from build123d import *

# Parameters (mm, degrees)
SKETCH1_R               = 2
BOSS_EXTRUDE1_DEPTH     = 2
FILLET1_R               = 7
SKETCH2_R               = 1.5
BOSS_EXTRUDE2_DEPTH     = 2.2
SKETCH3_R               = 1
BOSS_EXTRUDE3_DEPTH     = 2
SKETCH4_W               = 2
SKETCH4_H               = 15
BOSS_EXTRUDE4_DEPTH     = 7
FILLET3_START           = -3
FILLET3_DEPTH           = 6
FILLET3_2_DEPTH         = 2
FILLET3_START_2         = 1
FILLET3_3_DEPTH         = 2
CUT_EXTRUDE1_DEPTH      = 47.08088663
CUT_EXTRUDE1_DEPTH_BACK = 47.08088663
SKETCH5_R               = 2


with BuildPart() as part:
    # Sketch1 → Boss-Extrude1 (new body)
    with BuildSketch(Plane(origin=(0, 0, 0), x_dir=(1, 0, 0), z_dir=(0, 1, 0))):
        Polygon((-15, 0), (15, 0), (24.948794511, 37.5), (-24.948794511, 37.5), align=None)
        with Locations(Location((10, 26, 0), (0, 0, 270))):
            Circle(SKETCH1_R, mode=Mode.SUBTRACT)
        with Locations(Location((10, 6, 0), (0, 0, 270))):
            Circle(SKETCH1_R, mode=Mode.SUBTRACT)
        with Locations(Location((-10, 6, 0), (0, 0, 90))):
            Circle(SKETCH1_R, mode=Mode.SUBTRACT)
        with Locations(Location((-10, 26, 0), (0, 0, 90))):
            Circle(SKETCH1_R, mode=Mode.SUBTRACT)
    extrude(amount=BOSS_EXTRUDE1_DEPTH)

    # Fillet1
    fillet1_edges = [part.edges().sort_by_distance(p)[0] for p in [
        (-24.948794511, 1, -37.5),
        (24.948794511, 1, -37.5),
        (15, 1, 0),
        (-15, 1, 0),
    ]]
    fillet(fillet1_edges, radius=FILLET1_R)

    # Sketch2 → Boss-Extrude2 (add)
    with BuildSketch(Plane(origin=(0, 2, 0), x_dir=(1, 0, 0), z_dir=(0, 1, 0))):
        with Locations(Location((0, 34.5, 0), (0, 0, 270))):
            Circle(SKETCH2_R)
        with Locations(Location((18, 32.5, 0), (0, 0, 270))):
            Circle(SKETCH2_R)
        with Locations(Location((0, 4, 0), (0, 0, 270))):
            Circle(SKETCH2_R)
        with Locations(Location((0, 12, 0), (0, 0, 270))):
            Circle(SKETCH2_R)
        with Locations(Location((-18, 32.5, 0), (0, 0, 90))):
            Circle(SKETCH2_R)
    extrude(amount=BOSS_EXTRUDE2_DEPTH)

    # Sketch3 → Boss-Extrude3 (add)
    with BuildSketch(Plane(origin=(0, 4.2, 0), x_dir=(1, 0, 0), z_dir=(0, 1, 0))):
        with Locations(Location((-18, 32.5, 0), (0, 0, 270))):
            Circle(SKETCH3_R)
        with Locations(Location((0, 34.5, 0), (0, 0, 270))):
            Circle(SKETCH3_R)
        with Locations(Location((18, 32.5, 0), (0, 0, 270))):
            Circle(SKETCH3_R)
        with Locations(Location((0, 12, 0), (0, 0, 270))):
            Circle(SKETCH3_R)
        with Locations(Location((0, 4, 0), (0, 0, 270))):
            Circle(SKETCH3_R)
    extrude(amount=BOSS_EXTRUDE3_DEPTH)

    # Sketch4 → Boss-Extrude4 (add)
    with BuildSketch(Plane.XZ):
        with Locations((-2, -27)):
            Rectangle(SKETCH4_W, SKETCH4_H)
        with Locations((2, -27)):
            Rectangle(SKETCH4_W, SKETCH4_H)
    extrude(amount=BOSS_EXTRUDE4_DEPTH)

    # Fillet3: read off the stored shape, not the designer's step
    # Fillet3 outline → Fillet3 (cut)
    with BuildSketch(Plane.YZ.offset(FILLET3_START)):
        with BuildLine():
            Line((-7, -34.5), (-4, -34.5))
            ThreePointArc((-4, -34.5), (-6.121320344, -33.621320344), (-7, -31.5))
            Line((-7, -31.5), (-7, -34.5))
        make_face()
        with BuildLine():
            Line((-7, -19.5), (-7, -22.5))
            ThreePointArc((-7, -22.5), (-6.121320344, -20.378679656), (-4, -19.5))
            Line((-4, -19.5), (-7, -19.5))
        make_face()
    extrude(amount=FILLET3_DEPTH, mode=Mode.SUBTRACT)

    # Fillet3 2 outline → Fillet3 2 (add)
    with BuildSketch(Plane.YZ.offset(FILLET3_START)):
        with BuildLine():
            Line((0, -34.5), (-3, -34.5))
            ThreePointArc((-3, -34.5), (-0.878679656, -35.378679656), (0, -37.5))
            Line((0, -37.5), (0, -34.5))
        make_face()
        with BuildLine():
            Line((-3, -19.5), (0, -19.5))
            Line((0, -19.5), (0, -16.5))
            ThreePointArc((0, -16.5), (-0.878679656, -18.621320344), (-3, -19.5))
        make_face()
    extrude(amount=FILLET3_2_DEPTH)

    # Fillet3 3 outline → Fillet3 3 (add)
    with BuildSketch(Plane.YZ.offset(FILLET3_START_2)):
        with BuildLine():
            Line((0, -34.5), (-3, -34.5))
            ThreePointArc((-3, -34.5), (-0.878679656, -35.378679656), (0, -37.5))
            Line((0, -37.5), (0, -34.5))
        make_face()
        with BuildLine():
            Line((-3, -19.5), (0, -19.5))
            Line((0, -19.5), (0, -16.5))
            ThreePointArc((0, -16.5), (-0.878679656, -18.621320344), (-3, -19.5))
        make_face()
    extrude(amount=FILLET3_3_DEPTH)

    # Sketch5 → Cut-Extrude1 (cut, two sides: drawn at the far end of the back side and taken through both)
    with BuildSketch(Plane.ZY.offset(3).offset(-CUT_EXTRUDE1_DEPTH_BACK)):
        with Locations((-30.5, -3.5)):
            Circle(SKETCH5_R)
        with Locations((-23.5, -3.5)):
            Circle(SKETCH5_R)
    extrude(amount=CUT_EXTRUDE1_DEPTH + CUT_EXTRUDE1_DEPTH_BACK, mode=Mode.SUBTRACT)


solid = part.part
For this review, take the finished solid that the model builds, in its own axes (mm). A direction names the side the tool comes from. Round coordinates to 2 decimals unless told otherwise and drop trailing zeros. Loops run counter-clockwise (first coordinate to the right, second up) from the corner with the lowest first, then second, coordinate; pieces in that order, holes last. Notation, with made-up numbers: (2, 62.25) - (17, 62.25) arc R22 cw to (17, 96.25) - close; hole circle Ø9 at (4, 13.5). An arc over 180 degrees is marked (long way). Put each result on its own line as item: value. Start each with the question number.
1. Mouldability with a two-part tool opening along Z and no side actions: class faces 5 (the cylindrical face through (-21.45, 1.01, -34.7)), 6 (the cylindrical face through (0.45, 3.08, -2.57)), 7 (the cylindrical face through (1.99, -6.14, -20.4)) as +Z half, -Z half, draft (parallel to the pull), parting line (faces both ways), or undercut.
2. For faces 1 (the flat face through (0, 1, 0)), 2 (the flat face through (1, -4, -27)), 3 (the cylindrical face through (-0.9, 3.1, -35.7)), 4 (the flat face through (-2, -3.5, -34.5)), list the 3-axis set-ups (+Z, -Z, +X, -X, +Y, -Y) from which the entire face can be reached by the end or side of a thin tool; tool diameter is ignored.
3. Insertion check: P1, Ø4, axis at y = -1, z = -13.5, coming from the -X side; P2, Ø7.5, axis at y = -4.5, z = -23, coming from the +X side; P3, Ø3, axis at y = 0.5, z = -4.5, coming from the +X side; P4, Ø3, axis at x = -10, z = -6, coming from the -Y side. Each pin has a flat end and moves straight along its axis. Give the tip position at first contact, or say it passes through.
4. Consider section A-A on z = -30.5. State the section outline as (x, y) points.
5. Consider section B-B on y = 1. State the section outline as (x, z) points.
6. For probe 1 along Z at (x, y) = (2.5, -3.5); probe 2 along Z at (x, y) = (1, 2.5); probe 3 along X at (y, z) = (-5.5, -27), list the stretches that pass through material, from the lowest coordinate up. Write a range as [from, to].
7. Consider section D-D on x = 18. State the section outline as (y, z) points.
8. Consider section C-C on y = -3.5. State the section outline as (x, z) points.
Result sheet:
1. face 5: parting line
1. face 6: undercut
1. face 7: +Z half
2. face 1: +Z, +X, -X, +Y, -Y
2. face 2: +Z, -Z, -Y
2. face 3: +Y
2. face 4: -Z, +X, -X, -Y
3. P1: x = -19.04
3. P2: x = 3
3. P3: x = 16.59
3. P4: through
4. outline: (-22.85, 0) - (-3, 0) - (-3, -1.5) - (-1, -1.5) - (-1, 0) - (1, 0) - (1, -1.5) - (3, -1.5) - (3, 0) - (22.85, 0) - (22.85, 2) - (-22.85, 2) - close; (-3, -7) - (-1, -7) - (-1, -5.5) - (-3, -5.5) - close; (1, -7) - (3, -7) - (3, -5.5) - (1, -5.5) - close
5. outline: (-22.62, -28.7) arc R7 ccw to (-15.85, -37.5) - (15.85, -37.5) arc R7 ccw to (22.62, -28.7) - (16.38, -5.2) arc R7 ccw to (9.61, 0) - (-9.61, 0) arc R7 ccw to (-16.38, -5.2) - close; hole circle Ø4 at (-10, -26); hole circle Ø4 at (-10, -6); hole circle Ø4 at (10, -26); hole circle Ø4 at (10, -6)
6. probe 1: [-34.5, -32.5], [-28.5, -25.5], [-21.5, -19.5]
6. probe 2: [-35.62, -33.38], [-13.12, -10.88], [-5.12, -2.88]
6. probe 3: [-3, -1], [1, 3]
7. outline: (0, -37.16) - (2, -37.16) - (2, -34) - (4.2, -34) - (4.2, -33.5) - (6.2, -33.5) - (6.2, -31.5) - (4.2, -31.5) - (4.2, -31) - (2, -31) - (2, -11.31) - (0, -11.31) - close
8. outline: (-3, -34.5) - (-1, -34.5) - (-1, -32.5) - (-3, -32.5) - close; (-3, -28.5) - (-1, -28.5) - (-1, -25.5) - (-3, -25.5) - close; (-3, -21.5) - (-1, -21.5) - (-1, -19.5) - (-3, -19.5) - close; (1, -34.5) - (3, -34.5) - (3, -32.5) - (1, -32.5) - close; (1, -28.5) - (3, -28.5) - (3, -25.5) - (1, -25.5) - close; (1, -21.5) - (3, -21.5) - (3, -19.5) - (1, -19.5) - close
